from build123d import *
from OCP.BRepFilletAPI import BRepFilletAPI_MakeChamfer

# Parameters (mm, degrees)
SKETCH1_W           = 71.4
SKETCH1_H           = 30.1
BOSS_EXTRUDE1_DEPTH = 1.6
SKETCH4_W           = 47.2
SKETCH4_H           = 16
BOSS_EXTRUDE2_DEPTH = 17.4
SKETCH5_W           = 10.3
SKETCH5_H           = 10.3
BOSS_EXTRUDE3_DEPTH = 11
SKETCH6_W           = 7.8
SKETCH6_H           = 10
BOSS_EXTRUDE4_DEPTH = 10
SKETCH7_R           = 4
BOSS_EXTRUDE5_DEPTH = 16.5
SKETCH8_W           = 4
SKETCH8_H           = 12.8
CUT_EXTRUDE1_DEPTH  = 47.2
CUT_EXTRUDE2_DEPTH  = 10.3
CHAMFER1_SIZE       = 4
CHAMFER1_SIZE2      = 1.07179677


with BuildPart() as part:
    # Sketch1 → Boss-Extrude1 (new body)
    with BuildSketch(Plane(origin=(0, 0, 0), x_dir=(1, 0, 0), z_dir=(0, 1, 0))):
        Rectangle(SKETCH1_W, SKETCH1_H)
    extrude(amount=BOSS_EXTRUDE1_DEPTH)

    # Sketch4 → Boss-Extrude2 (add)
    with BuildSketch(Plane(origin=(0, 1.6, 0), x_dir=(1, 0, 0), z_dir=(0, 1, 0))):
        with Locations((-1.1, -4.05)):
            Rectangle(SKETCH4_W, SKETCH4_H)
    extrude(amount=BOSS_EXTRUDE2_DEPTH)

    # Sketch5 → Boss-Extrude3 (add)
    with BuildSketch(Plane(origin=(0, 1.6, 0), x_dir=(1, 0, 0), z_dir=(0, 1, 0))):
        with Locations((-30.35, 0)):
            Rectangle(SKETCH5_W, SKETCH5_H)
    extrude(amount=BOSS_EXTRUDE3_DEPTH)

    # Sketch6 → Boss-Extrude4 (add)
    with BuildSketch(Plane(origin=(0, 1.6, 0), x_dir=(1, 0, 0), z_dir=(0, 1, 0))):
        with Locations((32.4, 0)):
            Rectangle(SKETCH6_W, SKETCH6_H)
    extrude(amount=BOSS_EXTRUDE4_DEPTH)

    # Sketch7 → Boss-Extrude5 (add)
    with BuildSketch(Plane(origin=(0, 1.6, 0), x_dir=(1, 0, 0), z_dir=(0, 1, 0))):
        with Locations(Location((18.7, 10.55, 0), (0, 0, 90))):
            Circle(SKETCH7_R)
        with Locations(Location((10.2, 10.55, 0), (0, 0, 90))):
            Circle(SKETCH7_R)
        with Locations(Location((-18.7, 10.55, 0), (0, 0, 90))):
            Circle(SKETCH7_R)
    extrude(amount=BOSS_EXTRUDE5_DEPTH)

    # Sketch8 → Cut-Extrude1 (cut)
    with BuildSketch(Plane.ZY.offset(24.7)):
        with Locations((-0.95, 12.6)):
            Rectangle(SKETCH8_W, SKETCH8_H)
        with Locations((4.05, 12.6)):
            Rectangle(SKETCH8_W, SKETCH8_H)
        with Locations((9.05, 12.6)):
            Rectangle(SKETCH8_W, SKETCH8_H)
    extrude(amount=-CUT_EXTRUDE1_DEPTH, mode=Mode.SUBTRACT)

    # Sketch9 → Cut-Extrude2 (cut)
    with BuildSketch(Plane.XY.offset(5.15)):
        Polygon((-35.5, 12.6), (-35.5, 7.401794315), (-34.710010842, 8.059862443), (-33.280204433, 12.6), align=None)
        Polygon((-25.2, 12.6), (-26.836436424, 12.6), (-25.2, 6.114977788), align=None)
    extrude(amount=-CUT_EXTRUDE2_DEPTH, mode=Mode.SUBTRACT)

    # Chamfer1: one chamfer whose edges measure the first distance from different faces: ONE call of the kernel's chamfer builder (chamfer() names one face for all edges)
    chamfer1_edges_1 = [part.edges().sort_by_distance(p)[0] for p in [
        (36.3, 11.6, 0),
    ]]
    chamfer1_side_1 = [part.faces().sort_by_distance(p)[0] for p in [
        (36.3, 6.6, 0),
    ]]
    chamfer1_edges_2 = [part.edges().sort_by_distance(p)[0] for p in [
        (28.5, 11.6, 0),
    ]]
    chamfer1_side_2 = [part.faces().sort_by_distance(p)[0] for p in [
        (28.5, 6.6, 0),
    ]]
    chamfer1 = BRepFilletAPI_MakeChamfer(part.part.solid().wrapped)
    for e in chamfer1_edges_1:
        chamfer1.Add(CHAMFER1_SIZE, CHAMFER1_SIZE2, e.wrapped, chamfer1_side_1[0].wrapped)  # the first distance lies on this face
    for e in chamfer1_edges_2:
        chamfer1.Add(CHAMFER1_SIZE, CHAMFER1_SIZE2, e.wrapped, chamfer1_side_2[0].wrapped)  # the first distance lies on this face
    add(Compound.cast(chamfer1.Shape()), mode=Mode.REPLACE)


solid = part.part
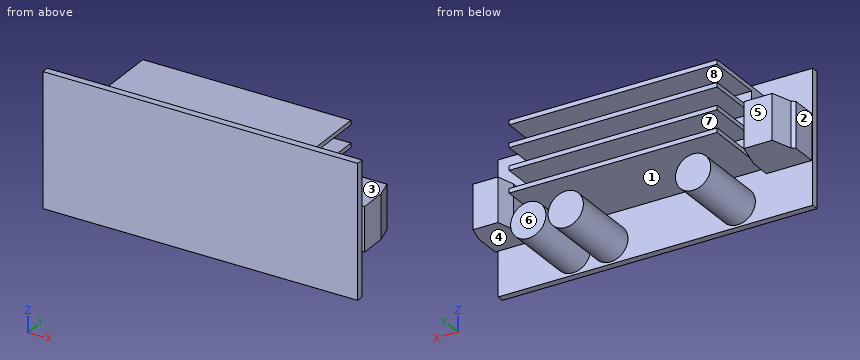
The listing builds one solid part. Answer for the finished solid, in the listing's coordinates (mm). Face numbers are marked on the shaded views. A direction names the side the tool comes from. Round coordinates to 2 decimals unless told otherwise and drop trailing zeros. Write each loop counter-clockwise with the first axis right and the second up, starting at its lowest first coordinate (ties: lowest second). Pieces come first, ordered by that corner, then holes. Notation, with made-up numbers: (21, 31) - (50, 31) arc R22 cw to (50, 66) - close; hole circle Ø10 at (87, 38.25). An arc over 180 degrees is marked (long way). Use a Markdown table: item, result. Add a question column.
1. A tool of negligible diameter and unlimited length cuts with its end or side. For the marked faces 4, 5, 6, 7 and 8, from which of +Z, -Z, +X, -X, +Y, -Y can it reach the whole face along a straight path? Write none if from no direction.
2. The part is cut by section D-D (y = 16.5). Write down the section's boundary in (x, z), and give its area (3 significant figures).
3. For a pull along Z with two mould halves and no side action, classify the marked faces 1, 2 and 3 as +Z half, -Z half, draft (parallel to the pull), parting line (faces both ways), or undercut.
4. Consider line 1 (Z direction, x = -19, y = 16.25); line 2 (Z direction, x = -13, y = 13.75); line 3 (X direction, y = 4.25, z = -2). Determine where each line is inside the solid, lowest interval first.
5. The part is cut by section C-C (z = -10.55). Write down the section's boundary in (x, y), and give its area (3 significant figures).
6. Flat-ended cylindrical pins translate along their axes: P1, Ø5, axis at x = -26, y = 14, coming from the +Z side; P2, Ø9, axis at x = 11, z = -10.5, coming from the +Y side; P3, Ø1.7, axis at y = 3.5, z = -2.5, coming from the -X side; P4, Ø2, axis at y = 16.5, z = 10, coming from the -X side. Find the tip coordinate at first contact, or state that the pin passes through.
7. The part is cut by section B-B (x = -9). Write down the section's boundary in (y, z), and give its area (3 significant figures).
8. The part is cut by section A-A (y = 3.5). Write down the section's boundary in (x, z).
Reported:
| question | item | result |
|---|---|---|
| 1 | face 4 | -Z, +X, +Y |
| 1 | face 5 | +Z, -Z, -X, +Y |
| 1 | face 6 | -Z, +X, -X, +Y |
| 1 | face 7 | +Y |
| 1 | face 8 | +X, -X, +Y |
| 2 | outline | (-24.7, -3.95) - (22.5, -3.95) - (22.5, -2.95) - (-24.7, -2.95) - close; (-24.7, 1.05) - (22.5, 1.05) - (22.5, 2.05) - (-24.7, 2.05) - close; (-24.7, 6.05) - (22.5, 6.05) - (22.5, 7.05) - (-24.7, 7.05) - close; (-24.7, 11.05) - (22.5, 11.05) - (22.5, 12.05) - (-24.7, 12.05) - close; circle Ø8 at (-18.7, -10.55); circle Ø8 at (10.2, -10.55); circle Ø8 at (18.7, -10.55) |
| 2 | area | 340 mm^2 |
| 3 | face 1 | undercut |
| 3 | face 2 | draft |
| 3 | face 3 | +Z half |
| 4 | line 1 | -14.54 to -6.56, -3.95 to -2.95, 1.05 to 2.05, 6.05 to 7.05, 11.05 to 12.05 |
| 4 | line 2 | -3.95 to -2.95, 1.05 to 2.05, 6.05 to 7.05, 11.05 to 12.05 |
| 4 | line 3 | -35.5 to -25.2, -24.7 to 22.5, 28.5 to 36.3 |
| 5 | outline | (-35.7, 0) - (35.7, 0) - (35.7, 1.6) - (22.7, 1.6) - (22.7, 18.1) - (14.7, 18.1) - (14.7, 1.6) - (14.2, 1.6) - (14.2, 18.1) - (6.2, 18.1) - (6.2, 1.6) - (-14.7, 1.6) - (-14.7, 18.1) - (-22.7, 18.1) - (-22.7, 1.6) - (-35.7, 1.6) - close |
| 5 | area | 510 mm^2 |
| 6 | P1 | z = 12.05 |
| 6 | P2 | y = 18.1 |
| 6 | P3 | x = -35.5 |
| 6 | P4 | through |
| 7 | outline | (0, -15.05) - (1.6, -15.05) - (1.6, -3.95) - (19, -3.95) - (19, -2.95) - (6.2, -2.95) - (6.2, 1.05) - (19, 1.05) - (19, 2.05) - (6.2, 2.05) - (6.2, 6.05) - (19, 6.05) - (19, 7.05) - (6.2, 7.05) - (6.2, 11.05) - (19, 11.05) - (19, 12.05) - (1.6, 12.05) - (1.6, 15.05) - (0, 15.05) - close |
| 7 | area | 173 mm^2 |
| 8 | outline | (-35.5, -5.15) - (-25.2, -5.15) - (-25.2, 5.15) - (-35.5, 5.15) - close; (-24.7, -3.95) - (22.5, -3.95) - (22.5, 12.05) - (-24.7, 12.05) - close; circle Ø8 at (-18.7, -10.55); circle Ø8 at (10.2, -10.55); circle Ø8 at (18.7, -10.55); (28.5, -5) - (36.3, -5) - (36.3, 5) - (28.5, 5) - close |
